For this review, take the finished solid that the model builds, in its own axes (mm). Coordinates: 2 decimals unless noted, no trailing zeros. Loops run counter-clockwise (first coordinate to the right, second up) from the corner with the lowest first, then second, coordinate; pieces in that order, holes last.
```python
from build123d import *

# Parameters (mm, degrees)
F0_W     = 40
F0_H     = 80
F1_DEPTH = 60
F2_R     = 5
F3_DEPTH = 40.001


with BuildPart() as f1:
    # F0 (on Top) → F1 (new body)
    with BuildSketch(Plane.XY):
        Rectangle(F0_W, F0_H)
    extrude(amount=-F1_DEPTH)

    # F2 (on face) → F3 (cut, through all)
    with BuildSketch(Plane.YZ.offset(20)):
        with Locations((20, -30.592106)):
            Circle(F2_R)
    extrude(amount=-F3_DEPTH, mode=Mode.SUBTRACT)


solid = f1.part
```
Q1. Consider section B-B (x = 1.5). State the section outline as (y, z) points.
Q2. Consider section A-A (y = 20). State the section outline as (x, z) points.
Q3. Wall thickness on probe 1 along Z at (x, y) = (7, 20); probe 2 along Z at (x, y) = (-5.5, 15.5): over which ranges is each line inside the solid? List them lowest first.
Q4. The part is to be moulded in two halves that separate along Y. For faces 1 (the face through (0, 40, -30)), 2 (the face through (0.28, 19.349, -25.635)), 3 (the face through (0, 1, 0)), say which applies: +Y half, -Y half, draft (parallel to the pull), parting line (faces both ways), or undercut.
Model answer:
1. outline: (-40, -60) - (40, -60) - (40, 0) - (-40, 0) - close; hole circle Ø10 at (20, -30.59)
2. outline: (-20, -60) - (20, -60) - (20, -35.59) - (-20, -35.59) - close; (-20, -25.59) - (20, -25.59) - (20, 0) - (-20, 0) - close
3. probe 1: z = -60 to -35.59, -25.59 to 0
3. probe 2: z = -60 to -32.77, -28.41 to 0
4. face 1: +Y half
4. face 2: undercut
4. face 3: draft
